Geometry: final body of the model. Coordinates: model frame, mm. A direction names the side the tool comes from. Round coordinates to 2 decimals unless told otherwise and drop trailing zeros. Loops run counter-clockwise (first coordinate to the right, second up) from the corner with the lowest first, then second, coordinate; pieces in that order, holes last. Notation, with made-up numbers: M -16.5,1 L 7.5,1 A11 ccw 7.5,7 Z; hole C 24,46 d8. An arc over 180 degrees is marked long. Answer as a JSON object with one key per item and string values.
from build123d import *

# Parameters (mm, degrees)
F0_W      = 16
F0_H      = 16
F1_DEPTH  = 16
F2_R      = 2
F4_DEPTH  = 1
F5_R      = 1.75
F6_DEPTH  = 1
F8_DEPTH  = 1
F10_DEPTH = 1
F11_R     = 1.75
F12_DEPTH = 1
F13_R     = 1.75
F14_DEPTH = 1


with BuildPart() as f1:
    # F0 (on Front) → F1 (new body)
    with BuildSketch(Plane.XZ):
        Rectangle(F0_W, F0_H)
    extrude(amount=F1_DEPTH)

    # F2
    f2_edges = [f1.edges().sort_by_distance(p)[0] for p in [
        (0, -16, 8),
        (-8, -8, 8),
        (8, -8, 8),
        (0, 0, 8),
        (0, 0, -8),
        (8, 0, 0),
        (-8, -8, -8),
        (-8, -16, 0),
        (-8, 0, 0),
        (0, -16, -8),
        (8, -16, 0),
        (8, -8, -8),
    ]]
    fillet(f2_edges, radius=F2_R)

    # F3 (on face) → F4 (cut)
    with BuildSketch(Plane.XZ.offset(16)):
        with BuildLine():
            Line((3, 1.25), (3, 3))
            Line((3, 3), (1.25, 3))
            ThreePointArc((1.25, 3), (1.7625631329, 1.7625631329), (3, 1.25))
        make_face()
        with BuildLine():
            Line((-3, -3), (-3, -1.25))
            ThreePointArc((-3, -1.25), (-4.2374368671, -4.2374368671), (-1.25, -3))
            Line((-1.25, -3), (-3, -3))
        make_face()
        with BuildLine():
            ThreePointArc((-1.25, -3), (-1.7625631329, -1.7625631329), (-3, -1.25))
            Line((-3, -1.25), (-3, -3))
            Line((-3, -3), (-1.25, -3))
        make_face()
        with BuildLine():
            Line((1.25, 3), (3, 3))
            Line((3, 3), (3, 1.25))
            ThreePointArc((3, 1.25), (4.2374368671, 1.7625631329), (4.75, 3))
            ThreePointArc((4.75, 3), (3, 4.75), (1.25, 3))
        make_face()
    extrude(amount=-F4_DEPTH, mode=Mode.SUBTRACT)

    # F5 (on face) → F6 (cut)
    with BuildSketch(Plane.XY.offset(8)):
        with BuildLine():
            Line((-3, -5), (-1.25, -5))
            ThreePointArc((-1.25, -5), (-4.2374368671, -3.7625631329), (-3, -6.75))
            Line((-3, -6.75), (-3, -5))
        make_face()
        with BuildLine():
            ThreePointArc((-3, -6.75), (-1.7625631329, -6.2374368671), (-1.25, -5))
            Line((-1.25, -5), (-3, -5))
            Line((-3, -5), (-3, -6.75))
        make_face()
        with BuildLine():
            Line((3, -11), (3, -9.25))
            ThreePointArc((3, -9.25), (1.7625631329, -9.7625631329), (1.25, -11))
            Line((1.25, -11), (3, -11))
        make_face()
        with BuildLine():
            ThreePointArc((4.75, -11), (4.2374368671, -9.7625631329), (3, -9.25))
            Line((3, -9.25), (3, -11))
            Line((3, -11), (1.25, -11))
            ThreePointArc((1.25, -11), (3, -12.75), (4.75, -11))
        make_face()
        with Locations((0, -8)):
            Circle(F5_R)
    extrude(amount=-F6_DEPTH, mode=Mode.SUBTRACT)

    # F7 (on face) → F8 (cut)
    with BuildSketch(Plane.YZ.offset(8)):
        with BuildLine():
            Line((-4.25, 3.75), (-6, 3.75))
            ThreePointArc((-6, 3.75), (-5.4874368671, 2.5125631329), (-4.25, 2))
            Line((-4.25, 2), (-4.25, 3.75))
        make_face()
        with BuildLine():
            ThreePointArc((-2.5, 3.75), (-4.25, 5.5), (-6, 3.75))
            Line((-6, 3.75), (-4.25, 3.75))
            Line((-4.25, 3.75), (-4.25, 2))
            ThreePointArc((-4.25, 2), (-3.0125631329, 2.5125631329), (-2.5, 3.75))
        make_face()
        with BuildLine():
            Line((-11.75, 3.75), (-10, 3.75))
            ThreePointArc((-10, 3.75), (-12.9874368671, 4.9874368671), (-11.75, 2))
            Line((-11.75, 2), (-11.75, 3.75))
        make_face()
        with BuildLine():
            ThreePointArc((-11.75, 2), (-10.5125631329, 2.5125631329), (-10, 3.75))
            Line((-10, 3.75), (-11.75, 3.75))
            Line((-11.75, 3.75), (-11.75, 2))
        make_face()
        with BuildLine():
            Line((-4.25, -3.75), (-4.25, -2))
            ThreePointArc((-4.25, -2), (-5.4874368671, -2.5125631329), (-6, -3.75))
            Line((-6, -3.75), (-4.25, -3.75))
        make_face()
        with BuildLine():
            ThreePointArc((-2.5, -3.75), (-3.0125631329, -2.5125631329), (-4.25, -2))
            Line((-4.25, -2), (-4.25, -3.75))
            Line((-4.25, -3.75), (-6, -3.75))
            ThreePointArc((-6, -3.75), (-4.25, -5.5), (-2.5, -3.75))
        make_face()
        with BuildLine():
            ThreePointArc((-10, -3.75), (-10.5125631329, -2.5125631329), (-11.75, -2))
            Line((-11.75, -2), (-11.75, -3.75))
            Line((-11.75, -3.75), (-10, -3.75))
        make_face()
        with BuildLine():
            Line((-11.75, -3.75), (-11.75, -2))
            ThreePointArc((-11.75, -2), (-12.9874368671, -4.9874368671), (-10, -3.75))
            Line((-10, -3.75), (-11.75, -3.75))
        make_face()
        with BuildLine():
            Line((-4.25, -1.75), (-4.25, 1.75))
            ThreePointArc((-4.25, 1.75), (-6, 0), (-4.25, -1.75))
        make_face()
        with BuildLine():
            ThreePointArc((-2.5, 0), (-3.0125631329, 1.2374368671), (-4.25, 1.75))
            Line((-4.25, 1.75), (-4.25, -1.75))
            ThreePointArc((-4.25, -1.75), (-3.0125631329, -1.2374368671), (-2.5, 0))
        make_face()
        with BuildLine():
            Line((-11.75, -1.75), (-11.75, 1.75))
            ThreePointArc((-11.75, 1.75), (-13.5, 0), (-11.75, -1.75))
        make_face()
        with BuildLine():
            ThreePointArc((-10, 0), (-10.5125631329, 1.2374368671), (-11.75, 1.75))
            Line((-11.75, 1.75), (-11.75, -1.75))
            ThreePointArc((-11.75, -1.75), (-10.5125631329, -1.2374368671), (-10, 0))
        make_face()
    extrude(amount=-F8_DEPTH, mode=Mode.SUBTRACT)

    # F9 (on face) → F10 (cut)
    with BuildSketch(Plane(origin=(0, 0, -8), x_dir=(1, 0, 0), z_dir=(0, 0, -1))):
        with BuildLine():
            Line((3, 11), (1.25, 11))
            ThreePointArc((1.25, 11), (1.7625631329, 9.7625631329), (3, 9.25))
            Line((3, 9.25), (3, 11))
        make_face()
        with BuildLine():
            ThreePointArc((4.75, 11), (3, 12.75), (1.25, 11))
            Line((1.25, 11), (3, 11))
            Line((3, 11), (3, 9.25))
            ThreePointArc((3, 9.25), (4.2374368671, 9.7625631329), (4.75, 11))
        make_face()
        with BuildLine():
            Line((-3, 11), (-1.25, 11))
            ThreePointArc((-1.25, 11), (-4.2374368671, 12.2374368671), (-3, 9.25))
            Line((-3, 9.25), (-3, 11))
        make_face()
        with BuildLine():
            ThreePointArc((-3, 9.25), (-1.7625631329, 9.7625631329), (-1.25, 11))
            Line((-1.25, 11), (-3, 11))
            Line((-3, 11), (-3, 9.25))
        make_face()
        with BuildLine():
            Line((3, 5), (3, 6.75))
            ThreePointArc((3, 6.75), (1.7625631329, 6.2374368671), (1.25, 5))
            Line((1.25, 5), (3, 5))
        make_face()
        with BuildLine():
            ThreePointArc((4.75, 5), (4.2374368671, 6.2374368671), (3, 6.75))
            Line((3, 6.75), (3, 5))
            Line((3, 5), (1.25, 5))
            ThreePointArc((1.25, 5), (3, 3.25), (4.75, 5))
        make_face()
        with BuildLine():
            ThreePointArc((-1.25, 5), (-1.7625631329, 6.2374368671), (-3, 6.75))
            Line((-3, 6.75), (-3, 5))
            Line((-3, 5), (-1.25, 5))
        make_face()
        with BuildLine():
            Line((-3, 5), (-3, 6.75))
            ThreePointArc((-3, 6.75), (-4.2374368671, 3.7625631329), (-1.25, 5))
            Line((-1.25, 5), (-3, 5))
        make_face()
    extrude(amount=-F10_DEPTH, mode=Mode.SUBTRACT)

    # F11 (on face) → F12 (cut)
    with BuildSketch(Plane(origin=(-8, 0, 0), x_dir=(0, -1, 0), z_dir=(-1, 0, 0))):
        with Locations((8, 0)):
            Circle(F11_R)
    extrude(amount=-F12_DEPTH, mode=Mode.SUBTRACT)

    # F13 (on face) → F14 (cut)
    with BuildSketch(Plane(origin=(0, 0, 0), x_dir=(-1, 0, 0), z_dir=(0, 1, 0))):
        with BuildLine():
            Line((3, 3), (1.25, 3))
            ThreePointArc((1.25, 3), (1.7625631329, 1.7625631329), (3, 1.25))
            Line((3, 1.25), (3, 3))
        make_face()
        with BuildLine():
            ThreePointArc((4.75, 3), (3, 4.75), (1.25, 3))
            Line((1.25, 3), (3, 3))
            Line((3, 3), (3, 1.25))
            ThreePointArc((3, 1.25), (4.2374368671, 1.7625631329), (4.75, 3))
        make_face()
        with BuildLine():
            Line((-3, 3), (-1.25, 3))
            ThreePointArc((-1.25, 3), (-4.2374368671, 4.2374368671), (-3, 1.25))
            Line((-3, 1.25), (-3, 3))
        make_face()
        with BuildLine():
            ThreePointArc((-3, 1.25), (-1.7625631329, 1.7625631329), (-1.25, 3))
            Line((-1.25, 3), (-3, 3))
            Line((-3, 3), (-3, 1.25))
        make_face()
        with BuildLine():
            Line((3, -3), (3, -1.25))
            ThreePointArc((3, -1.25), (1.7625631329, -1.7625631329), (1.25, -3))
            Line((1.25, -3), (3, -3))
        make_face()
        with BuildLine():
            ThreePointArc((4.75, -3), (4.2374368671, -1.7625631329), (3, -1.25))
            Line((3, -1.25), (3, -3))
            Line((3, -3), (1.25, -3))
            ThreePointArc((1.25, -3), (3, -4.75), (4.75, -3))
        make_face()
        with BuildLine():
            ThreePointArc((-1.25, -3), (-1.7625631329, -1.7625631329), (-3, -1.25))
            Line((-3, -1.25), (-3, -3))
            Line((-3, -3), (-1.25, -3))
        make_face()
        with BuildLine():
            Line((-3, -3), (-3, -1.25))
            ThreePointArc((-3, -1.25), (-4.2374368671, -4.2374368671), (-1.25, -3))
            Line((-1.25, -3), (-3, -3))
        make_face()
        Circle(F13_R)
    extrude(amount=-F14_DEPTH, mode=Mode.SUBTRACT)


solid = f1.part
1) Reachability of faces 1 (the flat face through (3, -1, 3)), 2 (the flat face through (7, -12, 0)), 3 (the flat face through (-3, -15, -3)), 4 (the cylindrical face through (1.617, -8.67, 7.507)), 5 (the flat face through (-7, -8, 0)) from +Z, -Z, +X, -X, +Y, -Y: full face, straight path, thin tool, end or side. Return the list, or none.
Results:
{"face 1": "+Y", "face 2": "+X", "face 3": "-Y", "face 4": "+Z", "face 5": "-X"}
2) Ray query, line 1 (Z direction, x = 3, y = -0.7); line 2 (Z direction, x = 7.25, y = -11); line 3 (Y direction, x = -3, z = -7.2). Return the intervals inside material, ascending.
Results:
{"line 1": "-7.52 to -4.75, -1.25 to 1.25, 4.75 to 7.52", "line 2": "-7.56 to -5.33, -2.17 to -1.58, 1.58 to 2.17, 5.33 to 7.56", "line 3": "-15.6 to -12.75, -9.25 to -6.75, -3.25 to -0.4"}
3) Section query D-D (z = 5). Return the cut outline in (x, y).
Results:
{"outline": "M -8,-14 A2 ccw -6,-16 L 6,-16 A2 ccw 8,-14 L 8,-12.97 L 7,-12.97 L 7,-10.53 L 8,-10.53 L 8,-5.47 L 7,-5.47 L 7,-3.03 L 8,-3.03 L 8,-2 A2 ccw 6,0 L -6,0 A2 ccw -8,-2 Z"}
4) Section query C-C (y = -3). Return the cut outline in (x, z).
Results:
{"outline": "M -8,-6 A2 ccw -6,-8 L 6,-8 A2 ccw 8,-6 L 8,-4.97 L 7,-4.97 L 7,-2.53 L 8,-2.53 L 8,-1.22 L 7,-1.22 L 7,1.22 L 8,1.22 L 8,2.53 L 7,2.53 L 7,4.97 L 8,4.97 L 8,6 A2 ccw 6,8 L -6,8 A2 ccw -8,6 Z"}
5) Section query A-A (x = 0). Return the cut outline in (y, z).
Results:
{"outline": "M -16,-6 A2 ccw -14,-8 L -2,-8 A2 ccw 0,-6 L 0,-1.75 L -1,-1.75 L -1,1.75 L 0,1.75 L 0,6 A2 ccw -2,8 L -6.25,8 L -6.25,7 L -9.75,7 L -9.75,8 L -14,8 A2 ccw -16,6 Z"}
6) Pin query (flat end, axial travel): P1, Ø1.1, axis at x = -3.5, z = -3.5, coming from the -Y side; P2, Ø4, axis at x = 0.5, z = 2.5, coming from the +Y side; P3, Ø1, axis at x = 3, y = -4, coming from the -Z side; P4, Ø3, axis at x = -3, z = -3, coming from the +Y side. Return the tip coordinate at first contact, or that it passes through.
Results:
{"P1": "y = -15", "P2": "y = 0", "P3": "z = -7", "P4": "y = -1"}
7) Section query B-B (z = 2.5). Return the cut outline in (x, y).
Results:
{"outline": "M -8,-14 A2 ccw -6,-16 L 1.32,-16 L 1.32,-15 L 4.68,-15 L 4.68,-16 L 6,-16 A2 ccw 8,-14 L 8,-12.97 L 7,-12.97 L 7,-10.53 L 8,-10.53 L 8,-5.47 L 7,-5.47 L 7,-3.03 L 8,-3.03 L 8,-2 A2 ccw 6,0 L 4.68,0 L 4.68,-1 L 1.32,-1 L 1.32,0 L -1.32,0 L -1.32,-1 L -4.68,-1 L -4.68,0 L -6,0 A2 ccw -8,-2 Z"}
8) Pull-direction query (X, two-part tool) for faces 6 (the flat face through (0, -8, 7)), 7 (the flat face through (3, -5, -7)), 8 (the flat face through (-8, -6.6, -1.4)), 9 (the cylindrical face through (7.4, -8.08, -7.43)); classes: +X half, -X half, draft (parallel to the pull), parting line (faces both ways), or undercut.
Results:
{"face 6": "undercut", "face 7": "undercut", "face 8": "-X half", "face 9": "+X half"}
